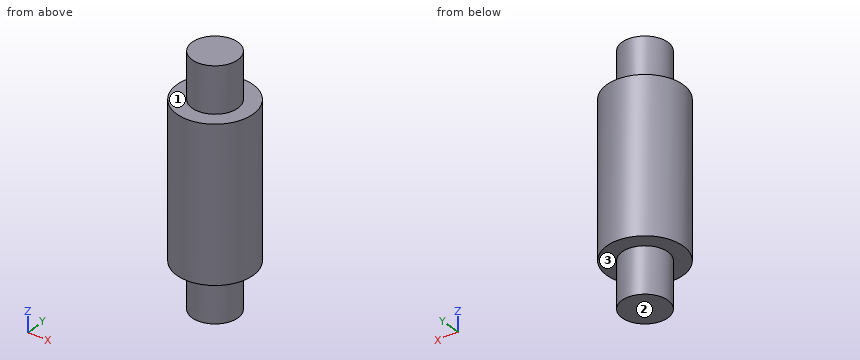
Autodesk Inventor part; units mm, degrees
ref_plane "YZ Plane" through (0, 0, 0) normal (1, 0, 0) x (0, 1, 0)
ref_plane "XZ Plane" through (0, 0, 0) normal (0, 1, 0) x (-1, 0, 0)
ref_plane "XY Plane" through (0, 0, 0) normal (0, 0, 1) x (1, 0, 0)
sketch "Sketch1" plane through (0, 0, 0) normal (0, 0, 1) x (1, 0, 0)
  circle A0 centre (0, 0) radius 2.5
  dimension "d0" = 5
extrude "Extrusion1" add sketch "Sketch1" along normal blind 10
sketch "Sketch2" plane through (0, 0, 10) normal (0, 0, 1) x (1, 0, 0)
  circle A0 centre (0, 0) radius 2.5
  circle A1 centre (0, 0) radius 1.5
  dimension "d3" = 3
extrude "Extrusion2" add sketch "Sketch2" along normal blind 3 contours A1
thread "Thread1"
sketch "Sketch3" plane through (0, 0, 0) normal (0, 0, -1) x (-1, 0, 0)
  circle A0 centre (0, 0) radius 2.5
  circle A1 centre (0, 0) radius 1.5
  dimension "d8" = 3
extrude "Extrusion3" add sketch "Sketch3" along normal blind 3 contours A1
thread "Thread2"
properties part number "spacer 1 cm"
The listing builds one solid part. Answer for the finished solid, in the listing's coordinates (mm). Face numbers are marked on the shaded views. A direction names the side the tool comes from. Give positions to 0.01 mm unless a question says otherwise; leave off trailing zeros. Order: outer loops, then holes, each group sorted by start corner. A loop starts at its lowest first (then second) coordinate and runs counter-clockwise, first axis right, second up. Notation, with made-up numbers: (-1.5, 6.25) -> (24.5, 6.25) arc R14 ccw to (24.5, 30.25) -> close; hole circle Ø3 at (-34, 42). An arc over 180 degrees is marked (long way). Answer as a JSON object with one key per item and string values. Group by question number.
Item 1: Flat-ended cylindrical pins translate along their axes: pin 1 (1.5 mm diameter, centred on x = -2, z = 4.5, fed in from -Y); pin 2 (3 mm diameter, centred on x = -2, z = 7, fed in from +Y). Find the tip coordinate at first contact, or state that the pin passes through.
Item 2: The part is cut by section A-A on y = 0. Write down the section's boundary in (x, z).
Item 3: A tool of negligible diameter and unlimited length cuts with its end or side. For the marked faces 1, 2 and 3, from which of +Z, -Z, +X, -X, +Y, -Y can it reach the whole face along a straight path? Write none if from no direction.
Item 4: The part is cut by section D-D on z = 12. Write down the section's boundary in (x, y).
Item 5: The part is cut by section C-C on z = 2.25. Write down the section's boundary in (x, y).
Item 6: Consider L1, parallel to Z at x = -1.4, y = 1.05; L2, parallel to X at y = 0.1, z = 8; L3, parallel to X at y = -0.1, z = 10.5. Determine where each line is inside the solid, lowest interval first. Write a range as from..to.
Result set:
{
 "1": {"pin 1": "y = -2.17", "pin 2": "y = 2.45"},
 "2": {"outline": "(-2.5, 0) -> (-1.5, 0) -> (-1.5, -3) -> (1.5, -3) -> (1.5, 0) -> (2.5, 0) -> (2.5, 10) -> (1.5, 10) -> (1.5, 13) -> (-1.5, 13) -> (-1.5, 10) -> (-2.5, 10) -> close"},
 "3": {"face 1": "+Z", "face 2": "-Z, +X, -X, +Y, -Y", "face 3": "-Z"},
 "4": {"outline": "circle Ø3 at (0, 0)"},
 "5": {"outline": "circle Ø5 at (0, 0)"},
 "6": {"L1": "0..10", "L2": "-2.5..2.5", "L3": "-1.5..1.5"}
}
